from build123d import *

# Parameters (mm, degrees)
F0_R            = 38.1
F1_DEPTH        = 50.8
F2_R            = 3.175
F3_DEPTH        = 6.35
F4_R            = 114.3
F5_DEPTH        = 6.35
F7_DEPTH        = 6.35
F7_COPIES_COUNT = 5
F7_COPIES_ANGLE = 240
F8_R            = 19.05
F9_DEPTH        = 6.35
F10_R           = 6.34999


# Not quite as in the source:
# - a fillet or chamfer is up to 0.001 mm smaller than in the source, because OpenCascade refuses the exact size
# - a pattern or mirror of a feature is missing from the dataset's text; its kind, count and spacing are read off the source's solid


with BuildPart() as f1:
    # F0 (on Top) → F1 (new body)
    with BuildSketch(Plane.XY):
        Circle(F0_R)
    extrude(amount=F1_DEPTH)

    # F2 (on face) → F3 (join)
    with BuildSketch(Plane(origin=(0, 0, 0), x_dir=(1, 0, 0), z_dir=(0, 0, -1))):
        Circle(F2_R)
    extrude(amount=F3_DEPTH)

    # F4 (on face) → F5 (join)
    with BuildSketch(Plane(origin=(0, 0, -6.35), x_dir=(1, 0, 0), z_dir=(0, 0, -1))):
        Circle(F4_R)
    extrude(amount=F5_DEPTH)

    # F6 (on face) → F7 (cut, through all)
    with BuildSketch(Plane(origin=(0, 0, -12.7), x_dir=(1, 0, 0), z_dir=(0, 0, -1))):
        with BuildLine():
            Line((16.880331728, 8.8293205148), (101.2819903679, 52.9759230889))
            ThreePointArc((101.2819903679, 52.9759230889), (98.9867036526, 57.15), (96.5194903679, 61.22481506))
            Line((96.5194903679, 61.22481506), (16.086581728, 10.2041358433))
            ThreePointArc((16.086581728, 10.2041358433), (16.4977839421, 9.525), (16.880331728, 8.8293205148))
        make_face()
        with BuildLine():
            ThreePointArc((96.5194903679, -61.22481506), (98.9867036526, -57.15), (101.2819903679, -52.9759230889))
            Line((101.2819903679, -52.9759230889), (16.880331728, -8.8293205148))
            ThreePointArc((16.880331728, -8.8293205148), (16.4977839421, -9.525), (16.086581728, -10.2041358433))
            Line((16.086581728, -10.2041358433), (96.5194903679, -61.22481506))
        make_face()
    f7 = extrude(amount=-F7_DEPTH, mode=Mode.SUBTRACT)

    # F7_copies: F7 ×5 about axis
    f7_copies_axis = Axis((0, 0, 0), (0, 0, 1))
    for i in range(1, F7_COPIES_COUNT):
        add(f7.rotate(f7_copies_axis, i * F7_COPIES_ANGLE / (F7_COPIES_COUNT - 1)), mode=Mode.SUBTRACT)

    # F8 (on face) → F9 (join)
    with BuildSketch(Plane(origin=(0, 0, -12.7), x_dir=(1, 0, 0), z_dir=(0, 0, -1))):
        Circle(F8_R)
    extrude(amount=F9_DEPTH)

    # F10 (radius 6.35 in the source; OpenCascade refuses exactly that, so slightly less here)
    f10_edges = [f1.edges().sort_by_distance(p)[0] for p in [
        (-19.05, 0, -19.05),
    ]]
    fillet(f10_edges, radius=F10_R)


solid = f1.part
Geometry check sheet. Reference: the model listing, model coordinates, mm. A direction names the side the tool comes from. Round coordinates to 2 decimals unless told otherwise and drop trailing zeros. Order: outer loops, then holes, each group sorted by start corner. A loop starts at its lowest first (then second) coordinate and runs counter-clockwise, first axis right, second up. Notation, with made-up numbers: (-2, 88.5) - (11, 88.5) arc R23 ccw to (11, 122.5) - close; hole circle Ø5 at (14, 4). An arc over 180 degrees is marked (long way). One line per question, with ' | ' between items. Start each with the question number.
(1) Release check for a two-part mould opening along Y. For faces 4 (the flat face through (56.866, -36.072, -9.569)), 5 (the flat face through (-77, -1, -12.7)), 6 (the cylindrical face through (-30.235, -23.183, 25.044)) record: released by +Y, released by -Y, zero draft, split by the parting line, or undercut.
(2) Sectioned sample at D-D on x = -29. Record the cut outline in (y, z), and give its area (3 significant figures).
(3) Thickness scan on L1, parallel to Z at x = -13, y = 14; L2, parallel to Y at x = -91.5, z = -12. Record the ranges inside material, lowest first. Write a range as [from, to].
(4) Sectioned sample at B-B on x = 53.5. Record the cut outline in (y, z).
(5) Depth check by flat-ended pin: pin 1 Ø2 at (x, y) = (74.5, 2.5) entering from +Z; pin 2 Ø5 at (x, y) = (-39, -69.5) entering from -Z; pin 3 Ø3 at (y, z) = (10, -7.5) entering from +X. Enter the tip coordinate at first touch or a pass-through.
(6) Sectioned sample at A-A on y = 83. Record the cut outline in (x, z), and give its area (3 significant figures).
(7) Access from +Z, -Z, +X, -X, +Y, -Y to the whole of each face (thin tool, end or side, straight path). Record for faces 1 (the flat face through (-59.67, -31.21, -9.57)), 2 (the flat face through (2.806, 67.283, -9.569)), 3 (the flat face through (2.75, -65.95, -9.57)).
Conclusion:
1) face 4: undercut | face 5: zero draft | face 6: split by the parting line
2) outline: (-110.56, -12.7) - (-18.4, -12.7) - (-18.4, -6.35) - (-110.56, -6.35) - close; (-24.71, 0) - (24.71, 0) - (24.71, 50.8) - (-24.71, 50.8) - close; (-15.17, -12.7) - (15.17, -12.7) - (15.17, -6.35) - (-15.17, -6.35) - close; (18.4, -12.7) - (110.56, -12.7) - (110.56, -6.35) - (18.4, -6.35) - close | area: 3,870 mm2
3) L1: z = [-12.7, -6.35], [0, 50.8] | L2: y = [-68.5, -58.04], [-47.86, 47.86], [58.04, 68.5]
4) outline: (-101.01, -12.7) - (-33.94, -12.7) - (-33.94, -6.35) - (-101.01, -6.35) - close; (-27.98, -12.7) - (27.98, -12.7) - (27.98, -6.35) - (-27.98, -6.35) - close; (33.94, -12.7) - (101.01, -12.7) - (101.01, -6.35) - (33.94, -6.35) - close
5) pin 1: stops at z = -6.35 | pin 2: stops at z = -12.7 | pin 3: stops at x = 113.98
6) outline: (-78.58, -12.7) - (-3.46, -12.7) - (-3.46, -6.35) - (-78.58, -6.35) - close; (3.46, -12.7) - (78.58, -12.7) - (78.58, -6.35) - (3.46, -6.35) - close | area: 954 mm2
7) face 1: -Z | face 2: -Z, +Y | face 3: -Z, -Y
